Autodesk Inventor part; units mm, degrees
ref_plane "YZ Plane" through (0, 0, 0) normal (1, 0, 0) x (0, 1, 0)
ref_plane "XZ Plane" through (0, 0, 0) normal (0, 1, 0) x (-1, 0, 0)
ref_plane "XY Plane" through (0, 0, 0) normal (0, 0, 1) x (1, 0, 0)
sketch "Sketch1" plane through (0, 0, 0) normal (0, 0, 1) x (1, 0, 0)
  circle A0 centre (0, 0) radius 20
  circle A1 centre (0, 0) radius 0.5
  dimension "d0" = 40
  dimension "d1" = 1
extrude "Extrusion1" add sketch "Sketch1" along normal blind 5
sketch "Sketch2" plane through (0, 0, 5) normal (0, 0, 1) x (1, 0, 0)
  circle A0 centre (0, 0) radius 0.5
  line L0 (0, 0) -> (0, 12.85)
  circle A1 centre (0, 12.85) radius 0.5
  line L1 (0, 0) -> (8.6813, 9.474)
  circle A2 centre (8.6813, 9.474) radius 0.5
  circle A3 centre (0, 0) radius 20
  line L2 (0, 0) -> (-20, 0)
  line L3 (0, 0) -> (20, 0) construction
  line L4 (0, 0) -> (-8.6813, -9.474)
  line L5 (0, 0) -> (12.85, 0) construction
  circle A4 centre (-8.6813, -9.474) radius 0.5
  line L6 (0, 0) -> (0, -12.85)
  circle A5 centre (0, -12.85) radius 0.5
  dimension "d4" = 12.85
  dimension "d5" = 1
  dimension "d6" = 12.85
  dimension "d8" = 1
  dimension "d15" = 90
  dimension "d17" = 47.5
  dimension "d18" = 42.5
  dimension "d20" = 12.85
  dimension "d21" = 132.5
  dimension "d22" = 1
  dimension "d23" = 12.85
  dimension "d24" = 1
  dimension "d25" = 42.5
extrude "Extrusion2" cut sketch "Sketch2" against normal blind 5 contours A5 | A4 | A1 | A2
properties part number "dondurgec"
Input: part model. Units: mm. Frame: model coordinates. Round coordinates to 2 decimals unless told otherwise and drop trailing zeros. Loops run counter-clockwise (first coordinate to the right, second up) from the corner with the lowest first, then second, coordinate; pieces in that order, holes last. Notation, with made-up numbers: (16, 52.25) -> (67, 52.25) arc R22 cw to (67, 67.25) -> close; hole circle Ø5 at (37.5, 45.5). An arc over 180 degrees is marked (long way). Write each question's results on one line, items separated by ' | '.
1. Section C-C (z = 2.55). Return loops of the section in (x, y).
Geometry results:
outline: circle Ø40 at (0, 0); hole circle Ø1 at (-8.68, -9.47); hole circle Ø1 at (0, -12.85); hole circle Ø1 at (0, 0); hole circle Ø1 at (0, 12.85); hole circle Ø1 at (8.68, 9.47)
2. Section B-B (x = 0). Return loops of the section in (y, z).
Geometry results:
outline: (-20, 0) -> (-13.35, 0) -> (-13.35, 5) -> (-20, 5) -> close; (-12.35, 0) -> (-0.5, 0) -> (-0.5, 5) -> (-12.35, 5) -> close; (0.5, 0) -> (12.35, 0) -> (12.35, 5) -> (0.5, 5) -> close; (13.35, 0) -> (20, 0) -> (20, 5) -> (13.35, 5) -> close
3. Ray query, line 1 (Y direction, x = 0, z = 1.05); line 2 (Y direction, x = 8.5, z = 4.85); line 3 (X direction, y = -13, z = 1.6). Return the intervals inside material, ascending. Write a range as from..to.
Geometry results:
line 1: -20..-13.35, -12.35..-0.5, 0.5..12.35, 13.35..20 | line 2: -18.1..9.01, 9.94..18.1 | line 3: -15.2..-0.48, 0.48..15.2
4. Section A-A (y = 0). Return loops of the section in (x, z).
Geometry results:
outline: (-20, 0) -> (-0.5, 0) -> (-0.5, 5) -> (-20, 5) -> close; (0.5, 0) -> (20, 0) -> (20, 5) -> (0.5, 5) -> close
5. Section D-D (y = 12.85). Return loops of the section in (x, z), and give its area (3 significant figures).
Geometry results:
outline: (-15.33, 0) -> (-0.5, 0) -> (-0.5, 5) -> (-15.33, 5) -> close; (0.5, 0) -> (15.33, 0) -> (15.33, 5) -> (0.5, 5) -> close | area: 148 mm2
6. First-contact query: P1, Ø3, axis at x = 1.5, z = 2, coming from the -Y side; P2, Ø8, axis at x = -4, y = 14, coming from the -Z side. Flat tips, straight axial feed; report the tip coordinate or a pass-through.
Geometry results:
P1: y = -20 | P2: z = 0
7. Mould query, pull axis Y, two halves, no side actions, for faces 1 (the face through (-0.108, 0.488, 2.465)), 2 (the face through (0, -4, 5)), 3 (the face through (-4.336, 19.524, 2.465)). Classes: +Y half, -Y half, draft (parallel to the pull), parting line (faces both ways), or undercut.
Geometry results:
face 1: undercut | face 2: draft | face 3: parting line
